from build123d import *

# Parameters (mm, degrees)
SKETCH1_W           = 25.4
SKETCH1_H           = 25.4
SKETCH1_W_2         = 22.225
SKETCH1_H_2         = 22.225
BOSS_EXTRUDE1_DEPTH = 850.9
SKETCH3_R           = 2.54
CUT_EXTRUDE2_DEPTH  = 852.657871448
SKETCH4_R           = 2.54
CUT_EXTRUDE3_DEPTH  = 852.657871448


with BuildPart() as part:
    # Sketch1 → Boss-Extrude1 (new body)
    with BuildSketch(Plane.XY):
        with Locations((12.7, 12.7)):
            Rectangle(SKETCH1_W, SKETCH1_H)
        with Locations((12.7, 12.7)):
            Rectangle(SKETCH1_W_2, SKETCH1_H_2, mode=Mode.SUBTRACT)
    extrude(amount=BOSS_EXTRUDE1_DEPTH)

    # Sketch3 → Cut-Extrude2 (cut, through all)
    with BuildSketch(Plane(origin=(0, 25.4, 0), x_dir=(1, 0, 0), z_dir=(0, 1, 0))):
        with Locations(Location((12.7, -812.8, 0), (0, 0, 90))):
            Circle(SKETCH3_R)
        with Locations(Location((12.7, -838.2, 0), (0, 0, 90))):
            Circle(SKETCH3_R)
        with Locations(Location((12.7, -12.7, 0), (0, 0, 270))):
            Circle(SKETCH3_R)
        with Locations(Location((12.7, -38.1, 0), (0, 0, 270))):
            Circle(SKETCH3_R)
        with Locations(Location((12.7, -63.5, 0), (0, 0, 270))):
            Circle(SKETCH3_R)
        with Locations(Location((6.35, -711.2, 0), (0, 0, 270))):
            Circle(SKETCH3_R)
        with Locations(Location((6.35, -685.8, 0), (0, 0, 270))):
            Circle(SKETCH3_R)
    extrude(amount=-CUT_EXTRUDE2_DEPTH, mode=Mode.SUBTRACT)

    # Sketch4 → Cut-Extrude3 (cut, through all)
    with BuildSketch(Plane(origin=(25.4, 0, 0), x_dir=(0, 0, -1), z_dir=(1, 0, 0))):
        with Locations((-793.75, 12.7)):
            Circle(SKETCH4_R)
        with Locations((-768.35, 12.7)):
            Circle(SKETCH4_R)
    extrude(amount=-CUT_EXTRUDE3_DEPTH, mode=Mode.SUBTRACT)


solid = part.part
Work out the finished part from the listing and answer in its coordinate system (mm). A direction names the side the tool comes from. Give positions to 0.01 mm unless a question says otherwise; leave off trailing zeros. Write each loop counter-clockwise with the first axis right and the second up, starting at its lowest first coordinate (ties: lowest second). Pieces come first, ordered by that corner, then holes.
Q1. A tool of negligible diameter and unlimited length cuts with its end or side. For faces 1 (the face through (13, 25.4, 419)), 2 (the face through (13, 1.587, 419)), from which of +Z, -Z, +X, -X, +Y, -Y can it reach the whole face along a straight path? Write none if from no direction.
Answer:
face 1: +Z, -Z, +X, -X, +Y
face 2: +Z, -Z
Q2. For a pull along X with two mould halves and no side action, classify faces 3 (the face through (1, 13, 850.9)), 4 (the face through (13, 23.812, 419)), 5 (the face through (0, 13, 419)) as released by +X, released by -X, zero draft, split by the parting line, or undercut.
Answer:
face 3: zero draft
face 4: undercut
face 5: released by -X
Q3. Given pin 1 (12 mm diameter, centred on x = 16.5, y = 14, fed in from -Z), flat-ended and moving along its own axis, determine where the tip first touches the part or whether it passes through.
Answer:
pin 1: passes through
Q4. Straight lines are drawn through the part: L1, parallel to Y at x = 4, z = 216; L2, parallel to X at y = 24.95, z = 63.5. For each, find the intervals that lie inside material, in ascending order.
Answer:
L1: y = 0 to 1.59, 23.81 to 25.4
L2: x = 0 to 10.16, 15.24 to 25.4
Q5. The part is cut by section A-A on z = 116.5. Give the vertices of the cut face in (x, y).
Answer:
outline: (0, 0) - (25.4, 0) - (25.4, 25.4) - (0, 25.4) - close; hole (1.59, 1.59) - (23.81, 1.59) - (23.81, 23.81) - (1.59, 23.81) - close
